Autodesk Inventor part; units mm, degrees
ref_plane "YZ Plane" through (0, 0, 0) normal (1, 0, 0) x (0, 1, 0)
ref_plane "XZ Plane" through (0, 0, 0) normal (0, 1, 0) x (-1, 0, 0)
ref_plane "XY Plane" through (0, 0, 0) normal (0, 0, 1) x (1, 0, 0)
ref_plane "Work Plane1" through (0, 0, 0) normal (0, 0, 1) x (1, 0, 0)
ref_plane "Work Plane2" through (0, 0, 0) normal (0, 0, 1) x (1, 0, 0)
sketch "Sketch2" plane through (0, 0, 0) normal (0, 0, 1) x (1, 0, 0)
  circle A0 centre (24, 55) radius 16
  circle A1 centre (49, 30) radius 4
  circle A2 centre (-1, 80) radius 4
  circle A3 centre (34, 30) radius 4
  circle A4 centre (49, 65) radius 4
  circle A5 centre (14, 80) radius 4
  circle A6 centre (-1, 45) radius 4
  circle A7 centre (-1, 65) radius 4
  circle A8 centre (34, 80) radius 4
  circle A9 centre (49, 45) radius 4
  circle A10 centre (14, 30) radius 4
  circle A11 centre (-1, 30) radius 4
  circle A12 centre (49, 80) radius 4
  arc A13 (54, -29) -> (50, -25) centre (50, -29) ccw
  line L0 (50, -25) -> (10, -25)
  arc A14 (6, -21) -> (10, -25) centre (10, -21) ccw
  line L1 (6, -21) -> (6, 21)
  arc A15 (10, 25) -> (6, 21) centre (10, 21) ccw
  line L2 (10, 25) -> (52, 25)
  line L3 (52, 25) -> (54, 27)
  line L4 (54, 27) -> (54, 83)
  line L5 (54, 83) -> (52, 85)
  line L6 (52, 85) -> (-4, 85)
  line L7 (-4, 85) -> (-6, 83)
  line L8 (-6, 83) -> (-6, -33)
  arc A16 (-6, -33) -> (-2, -37) centre (-2, -33) ccw
  line L9 (-2, -37) -> (50, -37)
  arc A17 (50, -37) -> (54, -33) centre (50, -33) ccw
  line L10 (54, -33) -> (54, -29)
  line L11 (54, 35.5093) -> (-6, 35.5093)
  line L12 (54, 27) -> (54, -29)
  circle A18 centre (33.5, 2.5) radius 17.5 construction
  circle A19 centre (33.5, -5.6473) radius 17.75
  point P0 (0, 0)
  dimension "d11" = 35.5
extrude "Extrusion2" add sketch "Sketch2" along normal blind 4 contours L10 A17 L9 A16 L8 L11 L4 L3 L2 A15 L1 A14 L0 A13 | A13 L0 A14 L1 A15 L2 L3 L12
sketch "Sketch3" plane through (0, 0, 0) normal (0, 0, -1) x (-1, 0, 0)
  circle A0 centre (-33.5, -5.6473) radius 17.75
  circle A1 centre (-33.5, -5.6473) radius 16
  point P0 (0, 0)
  point P1 (-33.5, 2.5)
  dimension "d12" = 32
extrude "Extrusion3" add sketch "Sketch3" against normal blind 0.6
properties part number "30_XY_Sample_arm_35mmadapter"
Input: part model. Units: mm. Frame: model coordinates. A direction names the side the tool comes from. Coordinates: 2 decimals unless noted, no trailing zeros. Write each loop counter-clockwise with the first axis right and the second up, starting at its lowest first coordinate (ties: lowest second). Pieces come first, ordered by that corner, then holes. Notation, with made-up numbers: M 23.25,83 L 67.25,83 A9 ccw 67.25,98 Z; hole C 2.25,41 d3. An arc over 180 degrees is marked long. Use one line per item in the form item = value.
Q1. Set-up query: faces 1 (the face through (43, 8, 0.6)), 2 (the face through (33.479, 26.034, 1.972)). Return all of +Z, -Z, +X, -X, +Y, -Y with unobstructed straight access to the full face (end or side cutting, diameter ignored); none if empty.
Answer below:
face_1 = +Z
face_2 = +Z, -Z
Q2. Section A-A (x = 14). Return loops of the section in (y, z).
Answer below:
outline = M -37,0 L 26,0 L 26,4 L -37,4 Z; M 34,0 L 35.51,0 L 35.51,4 L 34,4 Z
Q3. Section C-C (y = 1). Return loops of the section in (x, z).
Answer below:
outline = M -6,0 L 18.95,0 L 18.95,0.6 L 17.04,0.6 L 17.04,4 L -6,4 Z; M 48.05,0 L 54,0 L 54,4 L 49.96,4 L 49.96,0.6 L 48.05,0.6 Z
Q4. Section D-D (x = 33). Return loops of the section in (y, z), plus the area to 3 significant figures.
Answer below:
outline = M -37,0 L -21.64,0 L -21.64,0.6 L -23.39,0.6 L -23.39,4 L -37,4 Z; M 10.34,0 L 26.13,0 L 26.13,4 L 12.1,4 L 12.1,0.6 L 10.34,0.6 Z; M 33.87,0 L 35.51,0 L 35.51,4 L 33.87,4 Z
area = 119 mm²
Q5. Material intervals for probe 1 along Y at (x, z) = (34, 1.45); probe 2 along Y at (x, z) = (14, 2.75); probe 3 along Y at (x, z) = (33.5, 0.15), sorted ascending. Write a range as from..to.
Answer below:
probe_1 = -37..-23.39, 12.1..26, 34..35.51
probe_2 = -37..26, 34..35.51
probe_3 = -37..-21.65, 10.35..26.03, 33.97..35.51
Q6. Section B-B (z = 1.3). Return loops of the section in (x, y).
Answer below:
outline = M -6,-33 A4 ccw -2,-37 L 50,-37 A4 ccw 54,-33 L 54,35.51 L -6,35.51 Z; hole C -1,30 d8; hole C 14,30 d8; hole C 33.5,-5.65 d35.5; hole C 34,30 d8; hole C 49,30 d8
